```python
from build123d import *

# Parameters (mm, degrees)
SKETCH1_R           = 2.75
BOSS_EXTRUDE1_DEPTH = 105
SKETCH2_R           = 25
SKETCH2_R_2         = 7.920218335
BOSS_EXTRUDE2_DEPTH = 7
SKETCH3_R           = 25
SKETCH3_R_2         = 7
CUT_EXTRUDE1_DEPTH  = 6
SKETCH3_2_R         = 7
CUT_EXTRUDE2_DEPTH  = 34


with BuildPart() as part:
    # Sketch1 → Boss-Extrude1 (new body)
    with BuildSketch(Plane.XY):
        Polygon((-26.568542495, 30), (26.568542495, 30), (30, 26.568542495), (30, -26.568542495), (26.568542495, -30), (-26.568542495, -30), (-30, -26.568542495), (-30, 26.568542495), align=None)
        with Locations((24.748737342, -24.748737342)):
            Circle(SKETCH1_R, mode=Mode.SUBTRACT)
        with Locations((-24.748737342, -24.748737342)):
            Circle(SKETCH1_R, mode=Mode.SUBTRACT)
        with Locations((24.748737342, 24.748737342)):
            Circle(SKETCH1_R, mode=Mode.SUBTRACT)
        with Locations((-24.748737342, 24.748737342)):
            Circle(SKETCH1_R, mode=Mode.SUBTRACT)
    extrude(amount=BOSS_EXTRUDE1_DEPTH)

    # Sketch2 → Boss-Extrude2 (add)
    with BuildSketch(Plane.XY.offset(105)):
        Circle(SKETCH2_R)
        Circle(SKETCH2_R_2, mode=Mode.SUBTRACT)
    extrude(amount=BOSS_EXTRUDE2_DEPTH)

    # Sketch3 → Cut-Extrude1 (cut)
    with BuildSketch(Plane(origin=(0, 0, 0), x_dir=(-1, 0, 0), z_dir=(0, 0, -1))):
        Circle(SKETCH3_R)
        Circle(SKETCH3_R_2, mode=Mode.SUBTRACT)
    extrude(amount=-CUT_EXTRUDE1_DEPTH, mode=Mode.SUBTRACT)

    # Sketch3_2 → Cut-Extrude2 (cut)
    with BuildSketch(Plane(origin=(0, 0, 0), x_dir=(-1, 0, 0), z_dir=(0, 0, -1))):
        Circle(SKETCH3_2_R)
    extrude(amount=-CUT_EXTRUDE2_DEPTH, mode=Mode.SUBTRACT)


solid = part.part
```
Work out the finished part from the listing and answer in its coordinate system (mm). A direction names the side the tool comes from. Round coordinates to 2 decimals unless told otherwise and drop trailing zeros. Loops run counter-clockwise (first coordinate to the right, second up) from the corner with the lowest first, then second, coordinate; pieces in that order, holes last. Notation, with made-up numbers: M 13,2.5 L 57,2.5 A15 ccw 57,20.5 Z; hole C 13.25,70.25 d4. An arc over 180 degrees is marked long. One line per question, with ' | ' between items.
Q1. Each of these flat-tipped pins is pushed along its axis until it touches: pin 1 Ø15.5 at (x, y) = (-3, -0.5) entering from -Z; pin 2 Ø3.5 at (x, y) = (24.75, 24.75) entering from +Z. Where does it stop, or does it pass through?
Conclusion:
pin 1: stops at z = 6 | pin 2: passes through
Q2. Consider line 1 along Y through (x, z) = (-25, 15.5); line 2 along X through (y, z) = (-24, 77.5); line 3 along Y through (x, z) = (23, 15.5). Determine where each line is inside the solid, lowest interval first. Write a range as from..to.
Conclusion:
line 1: y = -30..-27.49, -22.01..22.01, 27.49..30 | line 2: x = -30..-27.39, -22.1..22.1, 27.39..30 | line 3: y = -30..-26.87, -22.63..22.63, 26.87..30
Q3. Find section D-D, the plane z = 97. Give the vertices of the cut face in (x, y), then the cut area to 3 significant figures.
Conclusion:
outline: M -30,-26.57 L -26.57,-30 L 26.57,-30 L 30,-26.57 L 30,26.57 L 26.57,30 L -26.57,30 L -30,26.57 Z; hole C -24.75,-24.75 d5.5; hole C -24.75,24.75 d5.5; hole C 24.75,-24.75 d5.5; hole C 24.75,24.75 d5.5 | area: 3,480 mm2
Q4. Find section B-B, the plane y = 0. Give the vertices of the cut face in (x, z).
Conclusion:
outline: M -30,0 L -25,0 L -25,6 L -7,6 L -7,34 L 7,34 L 7,6 L 25,6 L 25,0 L 30,0 L 30,105 L 25,105 L 25,112 L 7.92,112 L 7.92,105 L -7.92,105 L -7.92,112 L -25,112 L -25,105 L -30,105 Z
Q5. The mould has two halves that part along Y. Classify faces 1 (the flat face through (28.31, -28.26, 51.76)), 2 (the flat face through (0, 30, 52)), 3 (the cylindrical face through (26, 22.3, 51.8)): +Y half, -Y half, draft (parallel to the pull), parting line (faces both ways), or undercut.
Conclusion:
face 1: -Y half | face 2: +Y half | face 3: undercut
Q6. A tool of negligible diameter and unlimited length cuts with its end or side. For faces 4 (the flat face through (0, 0, 34)), 5 (the flat face through (27, 0, 105)), 6 (the flat face through (-6, 6, 112)), from which of +Z, -Z, +X, -X, +Y, -Y can it reach the whole face along a straight path? Write none if from no direction.
Conclusion:
face 4: -Z | face 5: +Z | face 6: +Z, +X, -X, +Y, -Y
Q7. Find section A-A, the plane x = 20. Give the vertices of the cut face in (y, z), then the cut area to 3 significant figures.
Conclusion:
outline: M -30,0 L -15,0 L -15,6 L 15,6 L 15,0 L 30,0 L 30,105 L 15,105 L 15,112 L -15,112 L -15,105 L -30,105 Z | area: 6,330 mm2
Q8. Find section C-C, the plane z = 23. Give the vertices of the cut face in (x, y), then the cut area to 3 significant figures.
Conclusion:
outline: M -30,-26.57 L -26.57,-30 L 26.57,-30 L 30,-26.57 L 30,26.57 L 26.57,30 L -26.57,30 L -30,26.57 Z; hole C -24.75,-24.75 d5.5; hole C -24.75,24.75 d5.5; hole C 0,0 d14; hole C 24.75,-24.75 d5.5; hole C 24.75,24.75 d5.5 | area: 3,330 mm2
